The model under review builds one solid part; all positions refer to its coordinate system, in mm. A direction names the side the tool comes from. Round coordinates to 2 decimals unless told otherwise and drop trailing zeros. Write each loop counter-clockwise with the first axis right and the second up, starting at its lowest first coordinate (ties: lowest second). Pieces come first, ordered by that corner, then holes. Notation, with made-up numbers: (-6, 71) - (33, 71) arc R33 cw to (33, 110) - close; hole circle Ø1 at (4, -21). An arc over 180 degrees is marked (long way). Write each question's results on one line, items separated by ' | '.
```python
from build123d import *

# Parameters (mm, degrees)
SKETCH1_R           = 4
BOSS_EXTRUDE1_DEPTH = 20
CUT_EXTRUDE1_DEPTH  = 10


with BuildPart() as part:
    # Sketch1 → Boss-Extrude1 (new body)
    with BuildSketch(Plane(origin=(0, 0, 0), x_dir=(1, 0, 0), z_dir=(0, 1, 0))):
        with Locations(Location((0, 0, 0), (0, 0, 270))):
            Circle(SKETCH1_R)
    extrude(amount=BOSS_EXTRUDE1_DEPTH)

    # Sketch2 → Cut-Extrude1 (cut)
    with BuildSketch(Plane(origin=(0, 20, 0), x_dir=(1, 0, 0), z_dir=(0, 1, 0))):
        with BuildLine():
            ThreePointArc((2.5, 2.5), (0, 1.464466094), (-2.5, 2.5))
            ThreePointArc((-2.5, 2.5), (-1.464466094, 0), (-2.5, -2.5))
            ThreePointArc((-2.5, -2.5), (0, -1.464466094), (2.5, -2.5))
            ThreePointArc((2.5, -2.5), (1.464466094, 0), (2.5, 2.5))
        make_face()
    extrude(amount=-CUT_EXTRUDE1_DEPTH, mode=Mode.SUBTRACT)


solid = part.part
```
Q1. For probe 1 along X at (y, z) = (11.25, -2); probe 2 along Y at (x, z) = (0.5, 0.5); probe 3 along X at (y, z) = (18, 0.5), list the stretches that pass through material, from the lowest coordinate up.
Evaluation:
probe 1: x = -3.46 to -2.08, -1.87 to 1.87, 2.08 to 3.46 | probe 2: y = 0 to 10 | probe 3: x = -3.97 to -1.5, 1.5 to 3.97
Q2. Tool access review of faces 5 (the flat face through (0, 10, 0)), 6 (the flat face through (0, 0, 0)): name each direction out of +Z, -Z, +X, -X, +Y, -Y from which nothing blocks a thin tool from reaching the whole face with its end or side.
Evaluation:
face 5: +Y | face 6: +Z, -Z, +X, -X, -Y
Q3. We need section D-D (y = 1.75). State the section outline as (x, z) points.
Evaluation:
outline: circle Ø8 at (0, 0)
Q4. We need section A-A (z = 0). State the section outline as (x, y) points, plus the area to 3 significant figures.
Evaluation:
outline: (-4, 0) - (4, 0) - (4, 20) - (1.46, 20) - (1.46, 10) - (-1.46, 10) - (-1.46, 20) - (-4, 20) - close | area: 131 mm^2
Q5. We need section C-C (x = 0). State the section outline as (y, z) points, plus the area to 3 significant figures.
Evaluation:
outline: (0, -4) - (20, -4) - (20, -1.46) - (10, -1.46) - (10, 1.46) - (20, 1.46) - (20, 4) - (0, 4) - close | area: 131 mm^2
Q6. The part is to be moulded in two halves that separate along X. For faces 1 (the flat face through (0, 20, 2)), 2 (the cylindrical face through (0.039, 15.07, -1.465)), 3 (the cylindrical face through (1.465, 15.07, 0.039)), 4 (the cylindrical face through (-3.905, 9.86, -0.867)), say which applies: released by +X, released by -X, zero draft, split by the parting line, or undercut.
Evaluation:
face 1: zero draft | face 2: undercut | face 3: undercut | face 4: split by the parting line
Q7. We need section B-B (y = 14). State the section outline as (x, z) points.
Evaluation:
outline: circle Ø8 at (0, 0); hole (-2.5, -2.5) arc R3.54 cw to (2.5, -2.5) arc R3.54 cw to (2.5, 2.5) arc R3.54 cw to (-2.5, 2.5) arc R3.54 cw to start
Q8. Insertion check: P1, Ø2, axis at y = 16, z = 1.5, coming from the +X side; P2, Ø4, axis at y = 8, z = 1, coming from the -X side. Each pin has a flat end and moves straight along its axis. Give the tip position at first contact, or say it passes through.
Evaluation:
P1: stops at x = 3.97 | P2: stops at x = -4
